For this review, use the dimensioned drawing (mm, ordinates from the lowest corner) and the shaded views. A direction names the side the tool comes from. Give positions to 0.01 mm unless a question says otherwise; leave off trailing zeros. Order: outer loops, then holes, each group sorted by start corner. A loop starts at its lowest first (then second) coordinate and runs counter-clockwise, first axis right, second up. Notation, with made-up numbers: (5.5, 21.25) -> (43.5, 21.25) arc R14 ccw to (43.5, 35.25) -> close; hole circle Ø9 at (5.25, 71.25). An arc over 180 degrees is marked (long way). Return JSON: item names as keys, results as strings.
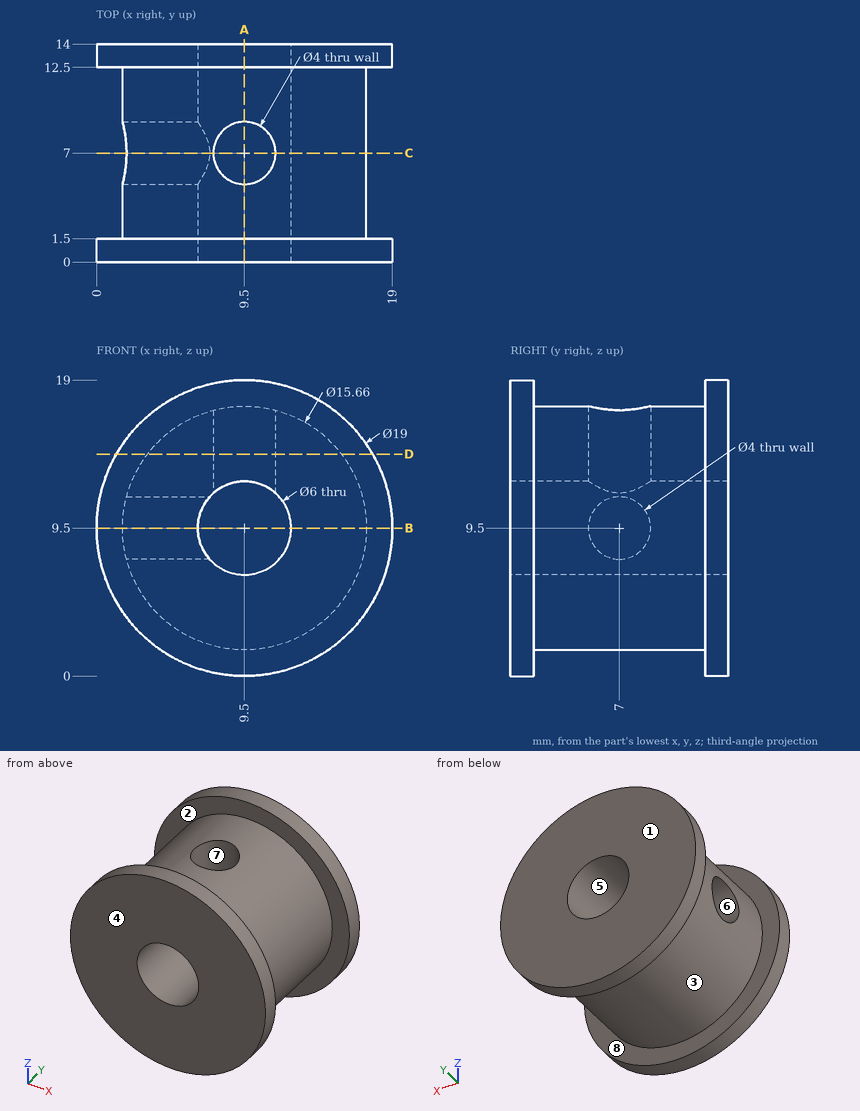
Item 1: For pin 1 (8 mm diameter, centred on x = 12, y = 7.5, fed in from -Z); pin 2 (1 mm diameter, centred on y = 9.5, z = 3.5, fed in from -X); pin 3 (5 mm diameter, centred on y = 5.5, z = 11, fed in from -X), all flat-tipped, find the tip position at first contact; note any pin that passes through.
Result set:
{"pin 1": "stops at z = 1.67", "pin 2": "stops at x = 3.93", "pin 3": "stops at x = 1.67"}
Item 2: Add section C-C (y = 7). Give the boundary of the cut face in (x, z), plus the area to 3 significant figures.
Result set:
{"outline": "(1.93, 7.5) arc R7.83 ccw (long way) to (11.5, 17.07) -> (11.5, 11.74) arc R3 cw (long way) to (7.26, 7.5) -> close; (1.93, 11.5) -> (7.26, 11.5) arc R3 cw to (7.5, 11.74) -> (7.5, 17.07) arc R7.83 ccw to start", "area": "124 mm^2"}
Item 3: Add section B-B (z = 9.5). Give the boundary of the cut face in (x, y).
Result set:
{"outline": "(0, 0) -> (6.5, 0) -> (6.5, 5) -> (1.67, 5) -> (1.67, 1.5) -> (0, 1.5) -> close; (0, 12.5) -> (1.67, 12.5) -> (1.67, 9) -> (6.5, 9) -> (6.5, 14) -> (0, 14) -> close; (12.5, 0) -> (19, 0) -> (19, 1.5) -> (17.33, 1.5) -> (17.33, 12.5) -> (19, 12.5) -> (19, 14) -> (12.5, 14) -> close"}
Item 4: Mouldability with a two-part tool opening along Y and no side actions: class the marked faces 1, 2, 3 and 4 as released by +Y, released by -Y, zero draft, split by the parting line, or undercut.
Result set:
{"face 1": "released by +Y", "face 2": "undercut", "face 3": "undercut", "face 4": "released by -Y"}
Item 5: Add section D-D (z = 14.25). Give the boundary of the cut face in (x, y), plus the area to 3 significant figures.
Result set:
{"outline": "(1.27, 0) -> (17.73, 0) -> (17.73, 1.5) -> (15.72, 1.5) -> (15.72, 12.5) -> (17.73, 12.5) -> (17.73, 14) -> (1.27, 14) -> (1.27, 12.5) -> (3.28, 12.5) -> (3.28, 1.5) -> (1.27, 1.5) -> close; hole circle Ø4 at (9.5, 7)", "area": "174 mm^2"}
Item 6: Add section A-A (x = 9.5). Give the boundary of the cut face in (y, z).
Result set:
{"outline": "(0, 0) -> (1.5, 0) -> (1.5, 1.67) -> (12.5, 1.67) -> (12.5, 0) -> (14, 0) -> (14, 6.5) -> (0, 6.5) -> close; (0, 12.5) -> (5, 12.5) -> (5, 17.33) -> (1.5, 17.33) -> (1.5, 19) -> (0, 19) -> close; (9, 12.5) -> (14, 12.5) -> (14, 19) -> (12.5, 19) -> (12.5, 17.33) -> (9, 17.33) -> close"}
Item 7: Machinability: for the marked faces 5, 6, 7 and 8, which of the approach directions +Z, -Z, +X, -X, +Y, -Y give a long, thin tool a straight path to every point of the face, cutting with its end or side? Answer none if there is none.
Result set:
{"face 5": "+Y, -Y", "face 6": "-X", "face 7": "+Z", "face 8": "none"}
Item 8: Wall thickness on L1, parallel to Y at x = 1.25, z = 8.25; L2, parallel to X at y = 3.75, z = 9.5; L3, parallel to Z at x = 9.5, y = 6.5: over which ranges is each line inside the solid? List them lowest first. Write a range as [from, to].
Result set:
{"L1": "y = [0, 1.5], [12.5, 14]", "L2": "x = [1.67, 6.5], [12.5, 17.33]", "L3": "z = [1.67, 6.5]"}
